from build123d import *

# Parameters (mm, degrees)
F0_R     = 2.75
F1_DEPTH = 3
F2_R     = 1.5
F3_DEPTH = 30
F4_SIZE  = 0.2
F6_DEPTH = 2
F7_R     = 0.4


with BuildPart() as f1:
    # F0 (on Front) → F1 (new body)
    with BuildSketch(Plane.XZ):
        Circle(F0_R)
    extrude(amount=F1_DEPTH)

    # F2 (on face) → F3 (join)
    with BuildSketch(Plane.XZ.offset(3)):
        Circle(F2_R)
    extrude(amount=F3_DEPTH)

    # F4
    f4_edges = [f1.edges().sort_by_distance(p)[0] for p in [
        (-1.5, -33, 0),
    ]]
    chamfer(f4_edges, length=F4_SIZE)

    # F5 (on face) → F6 (cut)
    with BuildSketch(Plane(origin=(0, 0, 0), x_dir=(-1, 0, 0), z_dir=(0, 1, 0))):
        Polygon((1.443376, 0), (0.721688, 1.25), (-0.721688, 1.25), (-1.443376, 0), (-0.721688, -1.25), (0.721688, -1.25), align=None)
    extrude(amount=-F6_DEPTH, mode=Mode.SUBTRACT)

    # F7
    f7_edges = [f1.edges().sort_by_distance(p)[0] for p in [
        (-2.75, 0, 0),
    ]]
    fillet(f7_edges, radius=F7_R)


solid = f1.part
Here's how the part is built. I have some questions about the finished solid (model axes, mm). A direction names the side the tool comes from. Round coordinates to 2 decimals unless told otherwise and drop trailing zeros. Order: outer loops, then holes, each group sorted by start corner. A loop starts at its lowest first (then second) coordinate and runs counter-clockwise, first axis right, second up. Notation, with made-up numbers: (79.25, 35.5) -> (104.25, 35.5) arc R18 ccw to (104.25, 43.5) -> close; hole circle Ø8 at (27, -39). An arc over 180 degrees is marked (long way). Return JSON: item names as keys, results as strings.
Q1. If we section it at B-B on y = -17: List the corners of the cut face in (x, z) for me, plus the area to 3 significant figures.
Filled sheet:
{"outline": "circle Ø3 at (0, 0)", "area": "7.07 mm^2"}
Q2. Which directions (+Z, -Z, +X, -X, +Y, -Y) give clear straight access to the entire face, cutting with the end or side of a thin tool? Please do faces 5 (the flat face through (0, 0, -2)), 6 (the flat face through (0, -1, 1.25)), 7 (the flat face through (1.2, -3, -1.2)).
Filled sheet:
{"face 5": "+Z, -Z, +X, -X, +Y", "face 6": "+Y", "face 7": "-Y"}
Q3. For pin 1 Ø1.5 at (y, z) = (-7.5, -1.5) entering from +X; pin 2 Ø3 at (x, y) = (0.5, -26.5) entering from +Z, each with a flat end and sliding along its axis, tell me the tip position at first contact or that it passes through.
Filled sheet:
{"pin 1": "stops at x = 1.3", "pin 2": "stops at z = 1.5"}
Q4. If we mould it in two halves opening along X, with no side actions, what happens to faces 1 (the cylindrical face through (-1.5, -17.69, 0.07)), 2 (the flat face through (1.08, -0.99, 0.63)), 3 (the flat face through (0, -1, -1.25)), 4 (the flat face through (0, -33, 0))? For each: released by +X, released by -X, zero draft, split by the parting line, or undercut.
Filled sheet:
{"face 1": "split by the parting line", "face 2": "undercut", "face 3": "undercut", "face 4": "zero draft"}
Q5. I need wall thicknesses on line 1 along X through (y, z) = (-10.5, 0.75); line 2 along Y through (x, z) = (-0.7, -0.1); line 3 along Y through (x, z) = (2.3, 0.6). Which ranges of each line are inside material? Lowest first, please. Write a range as from..to.
Filled sheet:
{"line 1": "x = -1.3..1.3", "line 2": "y = -33..-2", "line 3": "y = -3..0"}
Q6. If we section it at A-A on x = 0: List the corners of the cut face in (y, z) for me, plus the area to 3 significant figures.
Filled sheet:
{"outline": "(-33, -1.3) -> (-32.8, -1.5) -> (-3, -1.5) -> (-3, -2.75) -> (-0.4, -2.75) arc R0.4 ccw to (0, -2.35) -> (0, -1.25) -> (-2, -1.25) -> (-2, 1.25) -> (0, 1.25) -> (0, 2.35) arc R0.4 ccw to (-0.4, 2.75) -> (-3, 2.75) -> (-3, 1.5) -> (-32.8, 1.5) -> (-33, 1.3) -> close", "area": "101 mm^2"}
